For this review, use the dimensioned drawing (mm, ordinates from the lowest corner) and the shaded views. Coordinates: 2 decimals unless noted, no trailing zeros. Loops run counter-clockwise (first coordinate to the right, second up) from the corner with the lowest first, then second, coordinate; pieces in that order, holes last. Notation, with made-up numbers: (28.5, -15.75) - (48.5, -15.75) arc R20 cw to (48.5, 5.25) - close; hole circle Ø7 at (22.25, 43). An arc over 180 degrees is marked (long way). Answer in a Markdown table with one row per item. Add a question column.
(1) Mouldability with a two-part tool opening along Y and no side actions: class the marked faces 1 and 2 as +Y half, -Y half, draft (parallel to the pull), parting line (faces both ways), or undercut.
(2) We need section B-B on x = 130. Write out the cut boundary in (y, z), plus the area to 3 significant figures.
(3) We need section A-A on z = 83.5. Write out the cut boundary in (x, y), plus the area to 3 significant figures.
(4) For line 1 along Z through (x, y) = (660.4, 2.25) (1 decimal); line 2 along X through (y, z) = (2, 146.05) (1 decimal); line 3 along Z through (x, y) = (425.45, 2) (1 decimal), list the stretches that pass through material, from the lowest coordinate up.
(5) For P1, Ø3, axis at x = 632, y = 3.5, coming from the +Z side; P2, Ø3, axis at x = 144.5, y = 2.5, coming from the +Z side; P3, Ø3, axis at y = 2, z = 583.5, coming from the +X side, all flat-tipped, find the tip position at first contact; note any pin that passes through.
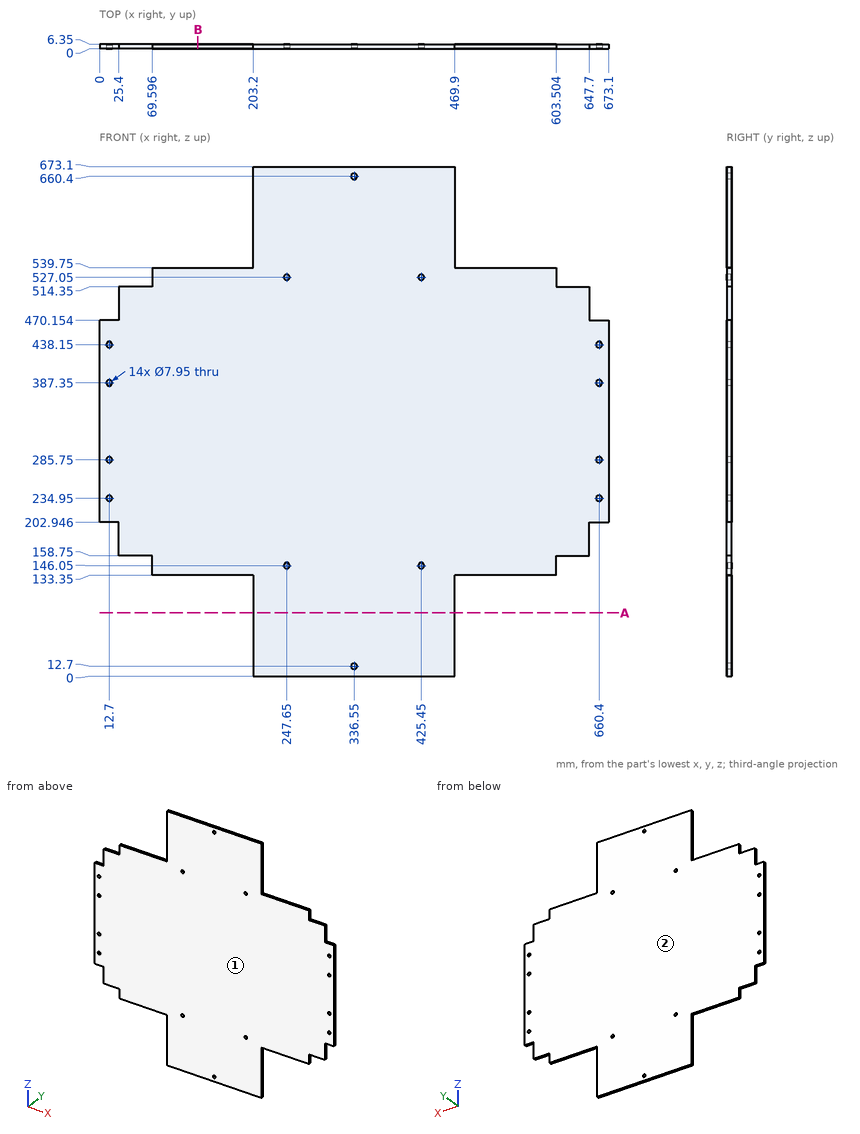
Outcome:
| question | item | result |
|---|---|---|
| 1 | face 1 | -Y half |
| 1 | face 2 | +Y half |
| 2 | outline | (0, 133.35) - (6.35, 133.35) - (6.35, 539.75) - (0, 539.75) - close |
| 2 | area | 2,580 mm² |
| 3 | outline | (203.2, 0) - (469.9, 0) - (469.9, 6.35) - (203.2, 6.35) - close |
| 3 | area | 1,690 mm² |
| 4 | line 1 | 202.9 to 231, 238.9 to 281.8, 289.7 to 383.4, 391.3 to 434.2, 442.1 to 470.2 |
| 4 | line 2 | 69.6 to 243.7, 251.6 to 421.5, 429.4 to 603.5 |
| 4 | line 3 | 0 to 142.1, 150 to 523.1, 531 to 673.1 |
| 5 | P1 | z = 514.35 |
| 5 | P2 | z = 539.75 |
| 5 | P3 | x = 469.9 |
